Build history of the part. All positions in model axes, mm. Face numbers are marked on the shaded views. Round coordinates to 2 decimals unless told otherwise and drop trailing zeros. Loops run counter-clockwise (first coordinate to the right, second up) from the corner with the lowest first, then second, coordinate; pieces in that order, holes last. Notation, with made-up numbers: (83.5, 16) - (139.5, 16) arc R11 cw to (139.5, 26) - close; hole circle Ø11 at (25.25, 31.5). An arc over 180 degrees is marked (long way). Use one line per item in the form item = value. Start each with the question number.
Q1. Drill centre lines: line 1 (X direction, y = 11.75, z = 0); line 2 (Z direction, x = -20.5, y = -4); line 3 (X direction, y = 2, z = 0). Where is each one in solid material? Low to high.
Q2. Saw through at A-A (x = -1). Give the cut face in (y, z).
Q3. Saw through at D-D (x = 26). Give the cut face in (y, z).
Q4. Pin check, flat tips, straight feed: pin 1 (3.5 mm diameter, centred on x = -20, z = -23, fed in from +Y); pin 2 (4 mm diameter, centred on x = -20, z = -29, fed in from -Y); pin 3 (1.3 mm diameter, centred on x = -19, z = 32.5, fed in from +Y); pin 4 (2.5 mm diameter, centred on x = -8.84, z = 8.84, fed in from +Y). Stop position of each tip, or through.
Q5. Saw through at B-B (y = 10.5). Give the cut face in (x, z), then the cut area to 3 significant figures.
Q6. Saw through at C-C (z = -23). Give the cut face in (x, y) (3 decimals), then the cut area to 3 significant figures.
Q7. Mould opens along X. For the marked faces 1, 2, 3 and 4 say: released by +X, released by -X, zero draft, split by the parting line, or undercut.
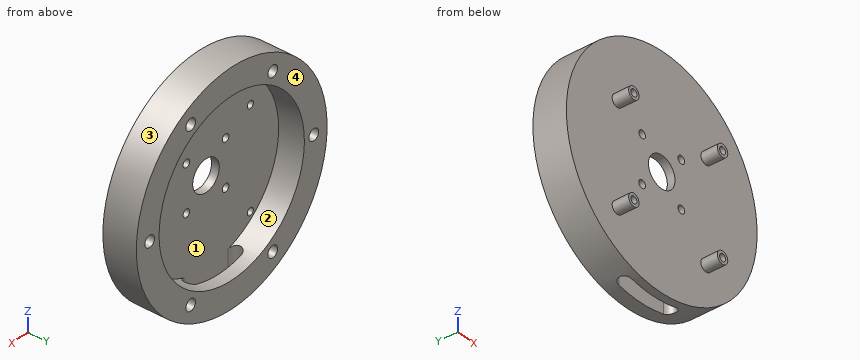
```python
from build123d import *

# Parameters (mm, degrees)
SKETCH_1_R          = 43
SKETCH_1_R_2        = 6
EXTRUDE_1_DEPTH     = 3
SKETCH_14_R         = 43
SKETCH_14_R_2       = 32.76
EXTRUDE_5_DEPTH     = 10
SKETCH_17_R         = 2.35
EXTRUDE_6_DEPTH     = 6.4
SKETCH_18_R         = 1.375
CUT_EXTRUDE_5_DEPTH = 64.83071361
SKETCH_23_R         = 2.2
CUT_EXTRUDE_6_DEPTH = 6.1
CUT_EXTRUDE1_DEPTH  = 20
SKETCH_26_R         = 1.5
CUT_EXTRUDE3_DEPTH  = 6.1
CIRPATTERN1_COUNT   = 4
CIRPATTERN2_COUNT   = 6


with BuildPart() as part:
    # 스케치1 → 보스-돌출1 (new body)
    with BuildSketch(Plane(origin=(0, 0, 0), x_dir=(1, 0, 0), z_dir=(0, 1, 0))):
        with Locations(Location((0, 0, 0), (0, 0, 270))):
            Circle(SKETCH_1_R)
        with Locations(Location((0, 0, 0), (0, 0, 270))):
            Circle(SKETCH_1_R_2, mode=Mode.SUBTRACT)
    extrude(amount=EXTRUDE_1_DEPTH)

    # 스케치14 → 보스-돌출5 (add)
    with BuildSketch(Plane(origin=(0, 3, 0), x_dir=(1, 0, 0), z_dir=(0, 1, 0))):
        with Locations(Location((0, 0, 0), (0, 0, 270))):
            Circle(SKETCH_14_R)
        with Locations(Location((0, 0, 0), (0, 0, 270))):
            Circle(SKETCH_14_R_2, mode=Mode.SUBTRACT)
    extrude(amount=EXTRUDE_5_DEPTH)

    # 스케치17 → 보스-돌출6 (add)
    with BuildSketch(Plane.XZ):
        with Locations(Location((20, 15, 0), (0, 0, 90))):
            Circle(SKETCH_17_R)
        with Locations(Location((-20, 15, 0), (0, 0, 90))):
            Circle(SKETCH_17_R)
        with Locations(Location((20, -23, 0), (0, 0, 90))):
            Circle(SKETCH_17_R)
        with Locations(Location((-20, -23, 0), (0, 0, 90))):
            Circle(SKETCH_17_R)
    extrude(amount=EXTRUDE_6_DEPTH)

    # 스케치18 → 컷-돌출5 (cut, through all)
    with BuildSketch(Plane.XZ.offset(6.4)):
        with Locations(Location((-20, 15, 0), (0, 0, 270))):
            Circle(SKETCH_18_R)
        with Locations(Location((20, 15, 0), (0, 0, 270))):
            Circle(SKETCH_18_R)
        with Locations(Location((20, -23, 0), (0, 0, 270))):
            Circle(SKETCH_18_R)
        with Locations(Location((-20, -23, 0), (0, 0, 270))):
            Circle(SKETCH_18_R)
    extrude(amount=-CUT_EXTRUDE_5_DEPTH, mode=Mode.SUBTRACT)

    # 스케치23 → 컷-돌출6 (cut)
    with BuildSketch(Plane(origin=(0, 13, 0), x_dir=(1, 0, 0), z_dir=(0, 1, 0))):
        with Locations(Location((18.5, 32.04293994, 0), (0, 0, 270))):
            Circle(SKETCH_23_R)
    cut_extrude_6 = extrude(amount=-CUT_EXTRUDE_6_DEPTH, mode=Mode.SUBTRACT)

    # Sketch2 → Cut-Extrude1 (cut)
    with BuildSketch(Plane(origin=(0, 0, -43), x_dir=(-1, 0, 0), z_dir=(0, 0, -1))):
        with BuildLine():
            Line((-10, 8), (10, 8))
            ThreePointArc((10, 8), (12.5, 5.5), (10, 3))
            Line((10, 3), (-10, 3))
            ThreePointArc((-10, 3), (-12.5, 5.5), (-10, 8))
        make_face()
    extrude(amount=-CUT_EXTRUDE1_DEPTH, mode=Mode.SUBTRACT)

    # 스케치26 → Cut-Extrude3 (cut)
    with BuildSketch(Plane(origin=(0, 3, 0), x_dir=(1, 0, 0), z_dir=(0, 1, 0))):
        with Locations(Location((8.838834765, 8.838834765, 0), (0, 0, 270))):
            Circle(SKETCH_26_R)
    cut_extrude3 = extrude(amount=-CUT_EXTRUDE3_DEPTH, mode=Mode.SUBTRACT)

    # CirPattern1: Cut-Extrude3 ×4 about axis
    cirpattern1_axis = Axis((0, 0, 0), (0, 1, 0))
    for i in range(1, CIRPATTERN1_COUNT):
        add(cut_extrude3.rotate(cirpattern1_axis, i * 360 / CIRPATTERN1_COUNT), mode=Mode.SUBTRACT)

    # CirPattern2: 컷-돌출6 ×6 about axis
    cirpattern2_axis = Axis((0, 0, 0), (0, 1, 0))
    for i in range(1, CIRPATTERN2_COUNT):
        add(cut_extrude_6.rotate(cirpattern2_axis, i * 360 / CIRPATTERN2_COUNT), mode=Mode.SUBTRACT)


solid = part.part
```
Report:
q1.line_1 = -43 to -39.2, -34.8 to -32.76, 32.76 to 34.8, 39.2 to 43
q1.line_2 = -25.3 to -24.28, -21.72 to -20.7, 12.7 to 13.72, 16.28 to 17.3
q1.line_3 = -43 to -6, 6 to 43
q2.outline = (0, -42.99) - (3, -42.99) - (3, -5.92) - (0, -5.92) - close; (0, 5.92) - (3, 5.92) - (3, 32.74) - (13, 32.74) - (13, 42.99) - (0, 42.99) - close; (8, -42.99) - (13, -42.99) - (13, -32.74) - (8, -32.74) - close
q3.outline = (0, -34.25) - (13, -34.25) - (13, -19.93) - (3, -19.93) - (3, 19.93) - (13, 19.93) - (13, 34.25) - (0, 34.25) - close
q4.pin_1 = 3
q4.pin_2 = 0
q4.pin_3 = 6.9
q4.pin_4 = through
q5.outline = circle Ø86 at (0, 0); hole circle Ø4.4 at (-37, 0); hole circle Ø65.52 at (0, 0); hole circle Ø4.4 at (-18.5, -32.04); hole circle Ø4.4 at (-18.5, 32.04); hole circle Ø4.4 at (18.5, -32.04); hole circle Ø4.4 at (18.5, 32.04); hole circle Ø4.4 at (37, 0)
q5.area = 2,350 mm²
q6.outline = (-36.332, 0) - (-22.35, 0) - (-22.35, -6.4) - (-21.375, -6.4) - (-21.375, 3) - (-23.328, 3) - (-23.328, 13) - (-36.332, 13) - close; (-18.625, -6.4) - (-17.65, -6.4) - (-17.65, 0) - (17.65, 0) - (17.65, -6.4) - (18.625, -6.4) - (18.625, 3) - (-18.625, 3) - close; (21.375, -6.4) - (22.35, -6.4) - (22.35, 0) - (36.332, 0) - (36.332, 13) - (23.328, 13) - (23.328, 3) - (21.375, 3) - close
q6.area = 487 mm²
q7.face_1 = undercut
q7.face_2 = undercut
q7.face_3 = split by the parting line
q7.face_4 = zero draft
